Part model, mm, in its own coordinate system. A direction names the side the tool comes from. Give positions to 0.01 mm unless a question says otherwise; leave off trailing zeros. Order: outer loops, then holes, each group sorted by start corner. A loop starts at its lowest first (then second) coordinate and runs counter-clockwise, first axis right, second up. Notation, with made-up numbers: (-35, 86) - (5, 86) arc R35 ccw to (5, 118) - close; hole circle Ø2 at (-17, -14.5). An arc over 180 degrees is marked (long way). Use one line per item in the form item = value. Start each with the question number.
1. Band-saw the part on B-B, the plane x = -31. List the corners of the cut face in (y, z).
2. Band-saw the part on D-D, the plane x = 19. List the corners of the cut face in (y, z), plus the area to 3 significant figures.
3. Tool access for faces 1 (the face through (-31, 3, -18.402)), 2 (the face through (28.402, 3, -21)), 3 (the face through (-29.753, 1.972, 21.517)): list every direction of +Z, -Z, +X, -X, +Y, -Y with a clear straight run to the whole face (end or side of a thin tool).
4. Pull direction X, two halves, no side cores. Call faces 4 (the face through (-28.402, 3, -21)), 5 (the face through (0, 0, -20)), 6 (the face through (-28.402, 3, 21)): +X half, -X half, draft (parallel to the pull), parting line (faces both ways), or undercut.
5. Band-saw the part on A-A, the plane y = 2.8. List the corners of the cut face in (x, z), plus the area to 3 significant figures.
6. Pin check, flat tips, straight feed: P1, Ø1.5, axis at x = 5.5, z = 21, coming from the +Y side; P2, Ø0.5, axis at y = 0.5, z = 2, coming from the -X side; P3, Ø0.5, axis at y = 0.5, z = 3, coming from the +X side. Stop position of each tip, or through.
7. Band-saw the part on C-C, the plane z = 21. List the corners of the cut face in (x, y).
8. Drill centre lines: line 1 (Z direction, x = 31, y = 1.75); line 2 (X direction, y = 2.65, z = 21); line 3 (Z direction, x = 15, y = 0.45). Where is each one in solid material? Low to high.
from build123d import *

# Parameters (mm, degrees)
SKETCH1_R           = 1.35
BOSS_EXTRUDE1_DEPTH = 4
SKETCH2_W           = 3
SKETCH2_H           = 36.803847578
SKETCH2_W_2         = 56.803847578
SKETCH2_H_2         = 3
CUT_EXTRUDE1_DEPTH  = 3


with BuildPart() as part:
    # Sketch1 → Boss-Extrude1 (new body)
    with BuildSketch(Plane(origin=(0, 0, 0), x_dir=(1, 0, 0), z_dir=(0, 1, 0))):
        with BuildLine():
            Line((-28.401923789, 22.5), (28.401923789, 22.5))
            ThreePointArc((28.401923789, 22.5), (33.121320344, 23.121320344), (32.5, 18.401923789))
            Line((32.5, 18.401923789), (32.5, -18.401923789))
            ThreePointArc((32.5, -18.401923789), (33.121320344, -23.121320344), (28.401923789, -22.5))
            Line((28.401923789, -22.5), (-28.401923789, -22.5))
            ThreePointArc((-28.401923789, -22.5), (-33.121320344, -23.121320344), (-32.5, -18.401923789))
            Line((-32.5, -18.401923789), (-32.5, 18.401923789))
            ThreePointArc((-32.5, 18.401923789), (-33.121320344, 23.121320344), (-28.401923789, 22.5))
        make_face()
        with Locations((31, 21)):
            Circle(SKETCH1_R, mode=Mode.SUBTRACT)
        with Locations((31, -21)):
            Circle(SKETCH1_R, mode=Mode.SUBTRACT)
        with Locations((-31, -21)):
            Circle(SKETCH1_R, mode=Mode.SUBTRACT)
        with Locations((-31, 21)):
            Circle(SKETCH1_R, mode=Mode.SUBTRACT)
        with BuildLine():
            Line((-28.401923789, 19.5), (28.401923789, 19.5))
            ThreePointArc((28.401923789, 19.5), (28.878679656, 18.878679656), (29.5, 18.401923789))
            Line((29.5, 18.401923789), (29.5, -18.401923789))
            ThreePointArc((29.5, -18.401923789), (28.878679656, -18.878679656), (28.401923789, -19.5))
            Line((28.401923789, -19.5), (-28.401923789, -19.5))
            ThreePointArc((-28.401923789, -19.5), (-28.878679656, -18.878679656), (-29.5, -18.401923789))
            Line((-29.5, -18.401923789), (-29.5, 18.401923789))
            ThreePointArc((-29.5, 18.401923789), (-28.878679656, 18.878679656), (-28.401923789, 19.5))
        make_face(mode=Mode.SUBTRACT)
    extrude(amount=BOSS_EXTRUDE1_DEPTH)

    # Sketch2 → Cut-Extrude1 (cut)
    with BuildSketch(Plane(origin=(0, 4, 0), x_dir=(1, 0, 0), z_dir=(0, 1, 0))):
        with Locations((-31, 0)):
            Rectangle(SKETCH2_W, SKETCH2_H)
        with Locations((0, -21)):
            Rectangle(SKETCH2_W_2, SKETCH2_H_2)
        with Locations((31, 0)):
            Rectangle(SKETCH2_W, SKETCH2_H)
        with Locations((0, 21)):
            Rectangle(SKETCH2_W_2, SKETCH2_H_2)
    extrude(amount=-CUT_EXTRUDE1_DEPTH, mode=Mode.SUBTRACT)


solid = part.part
From the geometry:
q1.outline = (0, -24) - (4, -24) - (4, -22.35) - (0, -22.35) - close; (0, -19.65) - (4, -19.65) - (4, -18.4) - (1, -18.4) - (1, 18.4) - (4, 18.4) - (4, 19.65) - (0, 19.65) - close; (0, 22.35) - (4, 22.35) - (4, 24) - (0, 24) - close
q2.outline = (0, -22.5) - (1, -22.5) - (1, -19.5) - (0, -19.5) - close; (0, 19.5) - (1, 19.5) - (1, 22.5) - (0, 22.5) - close
q2.area = 6.00 mm²
q3.face_1 = +X, -X, +Y
q3.face_2 = +Z, -Z, +Y
q3.face_3 = +Y, -Y
q4.face_4 = undercut
q4.face_5 = draft
q4.face_6 = undercut
q5.outline = (-32.5, -18.4) arc R3 ccw (long way) to (-28.4, -22.5) - (-28.4, -19.5) arc R3 ccw to (-29.5, -18.4) - close; (-32.5, 18.4) - (-29.5, 18.4) arc R3 ccw to (-28.4, 19.5) - (-28.4, 22.5) arc R3 ccw (long way) to start; (28.4, -22.5) arc R3 ccw (long way) to (32.5, -18.4) - (29.5, -18.4) arc R3 ccw to (28.4, -19.5) - close; (28.4, 19.5) arc R3 ccw to (29.5, 18.4) - (32.5, 18.4) arc R3 ccw (long way) to (28.4, 22.5) - close; hole circle Ø2.7 at (-31, -21); hole circle Ø2.7 at (-31, 21); hole circle Ø2.7 at (31, -21); hole circle Ø2.7 at (31, 21)
q5.area = 83.7 mm²
q6.P1 = 1
q6.P2 = -32.5
q6.P3 = 32.5
q7.outline = (-34, 0) - (-32.35, 0) - (-32.35, 4) - (-34, 4) - close; (-29.65, 0) - (29.65, 0) - (29.65, 4) - (28.4, 4) - (28.4, 1) - (-28.4, 1) - (-28.4, 4) - (-29.65, 4) - close; (32.35, 0) - (34, 0) - (34, 4) - (32.35, 4) - close
q8.line_1 = -24 to -22.35, -19.65 to -18.4, 18.4 to 19.65, 22.35 to 24
q8.line_2 = -34 to -32.35, -29.65 to -28.4, 28.4 to 29.65, 32.35 to 34
q8.line_3 = -22.5 to -19.5, 19.5 to 22.5
